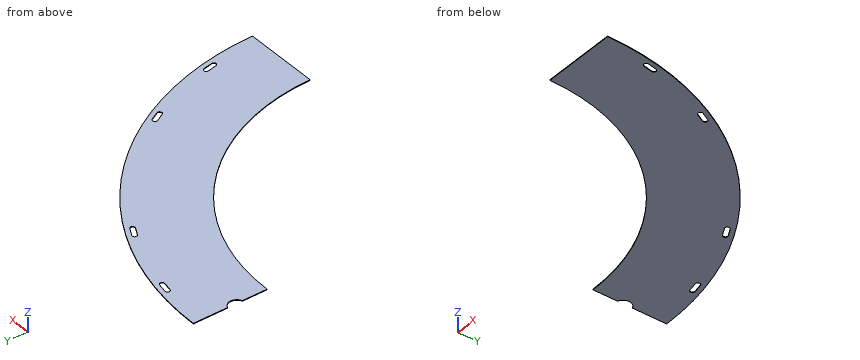
Autodesk Inventor part; units mm, degrees
ref_plane "YZ Plane" through (0, 0, 0) normal (1, 0, 0) x (0, 1, 0)
ref_plane "XZ Plane" through (0, 0, 0) normal (0, 1, 0) x (-1, 0, 0)
ref_plane "XY Plane" through (0, 0, 0) normal (0, 0, 1) x (1, 0, 0)
sketch "Sketch1" plane through (0, 0, 0) normal (0, 0, 1) x (1, 0, 0)
  arc A0 (187.325, 0) -> (0, 187.325) centre (0, 0) ccw
  arc A1 (136.525, 0) -> (0, 136.525) centre (0, 0) ccw
  line L0 (0, 136.525) -> (0, 187.325)
  line L1 (136.525, 0) -> (187.325, 0)
  point P0 (161.925, 0)
  point P1 (0, 161.925)
  dimension "d2" = 187.325
  dimension "d3" = 136.525
extrude "Extrusion1" add sketch "Sketch1" along normal blind 0.4
sketch "Sketch3" plane through (0, 0, 0.4) normal (0, 0, 1) x (1, 0, 0)
  arc A0 (178.117, 32.1925) -> (181.231, 32.8119) centre (179.674, 32.5022) ccw
  line L0 (178.117, 32.1925) -> (176.8782, 38.4205)
  arc A1 (179.9922, 39.0399) -> (176.8782, 38.4205) centre (178.4352, 38.7302) ccw
  line L1 (179.9922, 39.0399) -> (181.231, 32.8119)
  line L2 (160.9091, 89.6078) -> (163.9025, 84.0076)
  arc A2 (161.1024, 82.5109) -> (163.9025, 84.0076) centre (162.5024, 83.2593) ccw
  line L3 (161.1024, 82.5109) -> (158.109, 88.1111)
  arc A3 (160.9091, 89.6078) -> (158.109, 88.1111) centre (159.5091, 88.8595) ccw
  line L4 (84.0076, 163.9025) -> (89.6078, 160.9091)
  arc A4 (84.0076, 163.9025) -> (82.5109, 161.1024) centre (83.2593, 162.5024) ccw
  line L5 (88.1111, 158.109) -> (82.5109, 161.1024)
  arc A5 (88.1111, 158.109) -> (89.6078, 160.9091) centre (88.8595, 159.5091) ccw
  arc A6 (38.4205, 176.8782) -> (39.0399, 179.9922) centre (38.7302, 178.4352) ccw
  line L6 (32.8119, 181.231) -> (39.0399, 179.9922)
  arc A7 (32.8119, 181.231) -> (32.1925, 178.117) centre (32.5022, 179.674) ccw
  line L7 (38.4205, 176.8782) -> (32.1925, 178.117)
  circle A8 centre (-1.6445, 158.6401) radius 5.334
  point P0 (0, 0)
extrude "Extrusion2" cut sketch "Sketch3" against normal through all
properties part number "3DPRINT,CABLE,TRAY" material "ABS Plastic"
CAD build for the part. Positions are in the model's coordinates, mm. Give positions to 0.01 mm unless a question says otherwise; leave off trailing zeros. Loops run counter-clockwise (first coordinate to the right, second up) from the corner with the lowest first, then second, coordinate; pieces in that order, holes last. Notation, with made-up numbers: M 11.25,28.5 L 24.25,28.5 A22 ccw 24.25,35.5 Z; hole C 59.5,-25 d2. An arc over 180 degrees is marked long. Use one line per item in the form item = value.
Item 1: Slice it at C-C (x = 173). List the corners of the cut face in (y, z).
Determined:
outline = M 0,0 L 71.84,0 L 71.84,0.4 L 0,0.4 Z
Item 2: Slice it at A-A (z = 0.1). Count the separate pieces of the cut face and the enclosed holes in it, plus the area to 3 significant figures.
Determined:
separate_pieces = 1
enclosed_holes = 4
area = 12,800 mm2
Item 3: Drill centre lines: probe 1 along Y at (x, z) = (160.5, 0.2); probe 2 along Y at (x, z) = (171, 0.05); probe 3 along Y at (x, z) = (89, 0.3). Where is each one in solid material? Low to high. Write a range as from..to.
Determined:
probe_1 = 0..83.64, 90.1..96.59
probe_2 = 0..76.48
probe_3 = 103.53..157.93, 161.23..164.83
Item 4: Slice it at B-B (y = 13.5). List the corners of the cut face in (x, z), plus the area to 3 significant figures.
Determined:
outline = M 135.86,0 L 186.84,0 L 186.84,0.4 L 135.86,0.4 Z
area = 20.4 mm2
